from build123d import *

# Parameters (mm, degrees)
SKETCH1_W           = 154
SKETCH1_H           = 200
SKETCH1_W_2         = 140
SKETCH1_H_2         = 186
BOSS_EXTRUDE1_DEPTH = 5.5
FILLET1_R           = 5
SKETCH3_R           = 1.7
CUT_EXTRUDE1_DEPTH  = 127.329925196
CUT_EXTRUDE2_DEPTH  = 127.329925196
FILLET2_R           = 1


with BuildPart() as part:
    # Sketch1 → Boss-Extrude1 (new body)
    with BuildSketch(Plane(origin=(0, 0, 0), x_dir=(1, 0, 0), z_dir=(0, 1, 0))):
        Rectangle(SKETCH1_W, SKETCH1_H)
        Rectangle(SKETCH1_W_2, SKETCH1_H_2, mode=Mode.SUBTRACT)
    extrude(amount=BOSS_EXTRUDE1_DEPTH)

    # Fillet1
    fillet1_edges = [part.edges().sort_by_distance(p)[0] for p in [
        (70, 2.75, 93),
        (70, 2.75, -93),
        (-70, 2.75, -93),
        (-70, 2.75, 93),
        (-77, 2.75, -100),
        (77, 2.75, -100),
        (77, 2.75, 100),
        (-77, 2.75, 100),
    ]]
    fillet(fillet1_edges, radius=FILLET1_R)

    # Sketch3 → Cut-Extrude1 (cut, through all)
    with BuildSketch(Plane.XZ):
        with Locations(Location((73.5, -76.5, 0), (0, 0, 270))):
            Circle(SKETCH3_R)
        with Locations(Location((53.5, -96.5, 0), (0, 0, 270))):
            Circle(SKETCH3_R)
        with Locations(Location((-53.5, -96.5, 0), (0, 0, 270))):
            Circle(SKETCH3_R)
        with Locations(Location((-73.5, -76.5, 0), (0, 0, 270))):
            Circle(SKETCH3_R)
        with Locations(Location((-73.5, 0, 0), (0, 0, 270))):
            Circle(SKETCH3_R)
        with Locations(Location((-73.5, 76.5, 0), (0, 0, 270))):
            Circle(SKETCH3_R)
        with Locations(Location((-53.5, 96.5, 0), (0, 0, 270))):
            Circle(SKETCH3_R)
        with Locations(Location((53.5, 96.5, 0), (0, 0, 270))):
            Circle(SKETCH3_R)
        with Locations(Location((73.5, 76.5, 0), (0, 0, 270))):
            Circle(SKETCH3_R)
        with Locations(Location((73.5, 0, 0), (0, 0, 270))):
            Circle(SKETCH3_R)
        with Locations(Location((0, -96.5, 0), (0, 0, 270))):
            Circle(SKETCH3_R)
        with Locations(Location((0, 96.5, 0), (0, 0, 270))):
            Circle(SKETCH3_R)
    extrude(amount=-CUT_EXTRUDE1_DEPTH, mode=Mode.SUBTRACT)

    # Sketch4 → Cut-Extrude2 (cut, through all)
    with BuildSketch(Plane(origin=(0, 5.5, 0), x_dir=(1, 0, 0), z_dir=(0, 1, 0))):
        Polygon((-17.124355653, -100), (-5, -93), (-12, -93), (-24.124355653, -100), align=None)
    extrude(amount=-CUT_EXTRUDE2_DEPTH, mode=Mode.SUBTRACT)

    # Fillet2
    fillet2_edges = [part.edges().sort_by_distance(p)[0] for p in [
        (-17.124355653, 2.75, 100),
        (-24.124355653, 2.75, 100),
        (-12, 2.75, 93),
        (-5, 2.75, 93),
    ]]
    fillet(fillet2_edges, radius=FILLET2_R)


solid = part.part
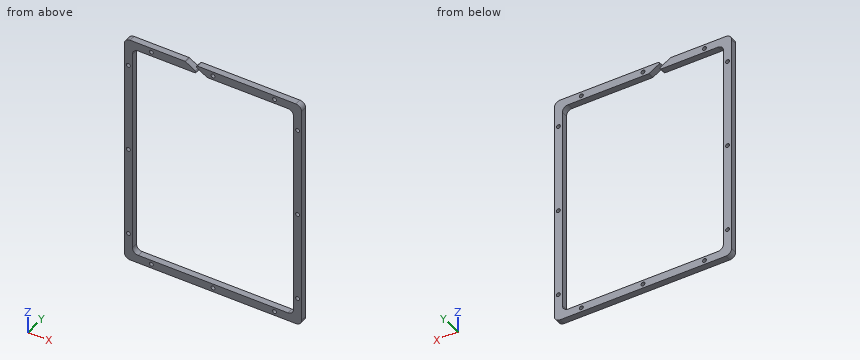
Source: CAD feature listing. Evaluate the final solid. Frame: model axes, mm. Coordinates: 2 decimals unless noted, no trailing zeros. Order: outer loops, then holes, each group sorted by start corner. A loop starts at its lowest first (then second) coordinate and runs counter-clockwise, first axis right, second up.
Item 1: Cut plane B-B (z = -34). Return loops of the section in (x, y).
Output values:
outline: (-77, 0) - (-70, 0) - (-70, 5.5) - (-77, 5.5) - close; (70, 0) - (77, 0) - (77, 5.5) - (70, 5.5) - close
Item 2: Material intervals for line 1 (X direction, y = 2.9, z = 76.5); line 2 (X direction, y = 1.8, z = -7); line 3 (Z direction, x = 9, y = 0.3), sorted ascending.
Output values:
line 1: x = -77 to -75.2, -71.8 to -70, 70 to 71.8, 75.2 to 77
line 2: x = -77 to -70, 70 to 77
line 3: z = -100 to -93, 93 to 100
Item 3: Cut plane A-A (x = -59). Return loops of the section in (y, z), plus the area to 3 significant figures.
Output values:
outline: (0, -100) - (5.5, -100) - (5.5, -93) - (0, -93) - close; (0, 93) - (5.5, 93) - (5.5, 100) - (0, 100) - close
area: 77.0 mm2
Item 4: Cut plane C-C (y = 1.4). Count the separate pieces of the cut face and the enclosed holes in it, plus the area to 3 significant figures.
Output values:
separate pieces: 1
enclosed holes: 12
area: 4,600 mm2
